Check sheet for the drawn part. Datum: minimum x, y, z corner. Units: mm. A direction names the side the tool comes from. Coordinates: 2 decimals unless noted, no trailing zeros. Return JSON: item names as keys, results as strings. Group by question number.
Q1. Go/stop test with a flat-tipped pin: pin 1 Ø1 at (x, z) = (6, 14) entering from +Y. Record where the tip stops, or that it passes through.
Q2. Access from +Z, -Z, +X, -X, +Y, -Y to the whole of each face (thin tool, end or side, straight path). Record for the marked faces 1, 2 and 3.
Q3. Thickness scan on probe 1 along Z at (x, y) = (9, 1.5); probe 2 along Z at (x, y) = (6.5, 9.75); probe 3 along X at (y, z) = (5.25, 19) (1 decimal). Record the ranges inside material, lowest first.
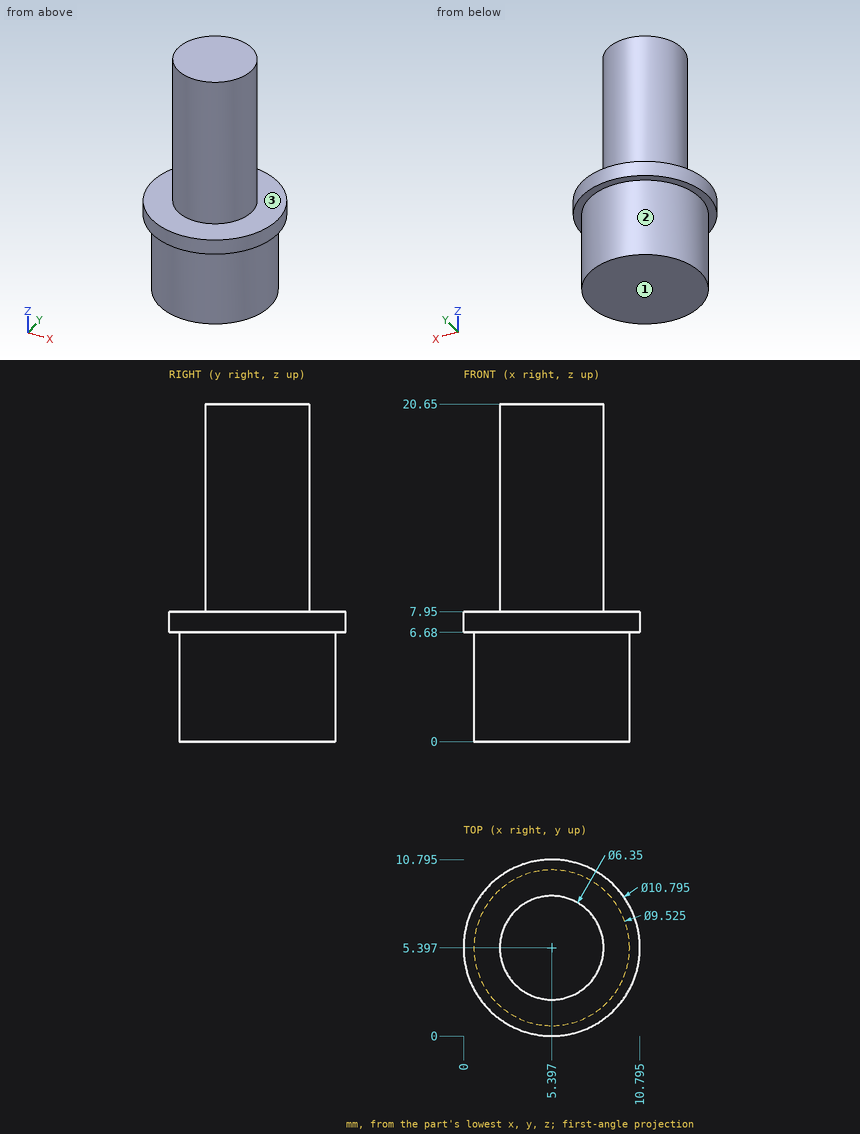
Numbers:
{
 "1": {"pin 1": "stops at y = 8.57"},
 "2": {"face 1": "-Z, +X, -X, +Y, -Y", "face 2": "-Z", "face 3": "+Z"},
 "3": {"probe 1": "z = 6.68 to 7.95", "probe 2": "z = 0 to 7.95", "probe 3": "x = 2.2 to 8.6"}
}
